The listing builds one solid part. Answer for the finished solid, in the listing's coordinates (mm). Round coordinates to 2 decimals unless told otherwise and drop trailing zeros. Order: outer loops, then holes, each group sorted by start corner. A loop starts at its lowest first (then second) coordinate and runs counter-clockwise, first axis right, second up. Notation, with made-up numbers: (43, 74.5) - (102, 74.5) arc R29 cw to (102, 102.5) - close; hole circle Ø8 at (1, 70.25). An arc over 180 degrees is marked (long way). One line per item, written item: value. Start each with the question number.
1. Section C-C, the plane y = 2 is taken. Give the vertices of the cut face in (x, z).
2. Section D-D, the plane z = -35 is taken. Give the vertices of the cut face in (x, y).
3. Section B-B, the plane x = -55 is taken. Give the vertices of the cut face in (y, z).
4. Section A-A, the plane x = -280 is taken. Give the vertices of the cut face in (y, z).
5. For a pull along Z with two mould halves and no side action, classify faces 1 (the flat face through (-150, 4, 0)), 2 (the flat face through (-145, 0, -25)), 3 (the flat face through (-145, 4, -50)), 4 (the cylindrical face through (-276.451, 4.563, -16.846)) as released by +Z, released by -Z, zero draft, split by the parting line, or undercut.
6. Straight lines are drawn through the part: line 1 (Z direction, x = -280, y = 4.5); line 2 (Z direction, x = -97.5, y = 5.5); line 3 (Z direction, x = -250, y = 3). For each, find the intervals that lie inside material, in ascending order.
7. A flat-ended cylindrical pin translates along its axis: P1, Ø6.5, axis at x = -280, z = -15, coming from the +Y side (3 decimals). Find the tip coordinate at first contact, or state that the pin passes through.
Autodesk Inventor part; units mm, degrees
ref_plane "YZ Plane" through (0, 0, 0) normal (1, 0, 0) x (0, 1, 0)
ref_plane "XZ Plane" through (0, 0, 0) normal (0, 1, 0) x (-1, 0, 0)
ref_plane "XY Plane" through (0, 0, 0) normal (0, 0, 1) x (1, 0, 0)
sketch "Skizze1" plane through (0, 0, 0) normal (0, 1, 0) x (-1, 0, 0)
  line L0 (0, 0) -> (275, 0)
  line L1 (275, 0) -> (275, -50)
  line L2 (275, -50) -> (0, -50)
  line L3 (0, -50) -> (0, 0)
  line L4 (275, 0) -> (275, -25)
  line L5 (275, -25) -> (250, -25)
  circle A0 centre (250, -25) radius 15
  line L6 (275, -50) -> (295, -50)
  line L7 (295, -50) -> (295, 0)
  line L8 (295, 0) -> (275, 0)
  dimension "d0" = 275
  dimension "d1" = 50
  dimension "d2" = 25
  dimension "d3" = 30
  dimension "d18" = 20
extrude "Extrusion1" add sketch "Skizze1" along normal blind 9 contours L0 L1 L2 L3
sketch "Skizze2" plane through (0, 9, 0) normal (0, 1, 0) x (1, 0, 0)
  line L0 (0, 0) -> (0, 50)
  line L1 (0, 50) -> (-30, 50)
  line L2 (-30, 50) -> (-30, 35)
  line L3 (0, 0) -> (-55, 0)
  line L4 (-275, 0) -> (0, 0)
  line L5 (-55, 0) -> (-70, 0)
  line L6 (-70, 0) -> (-55, 0)
  line L7 (-55, 0) -> (-55, 15)
  dimension "d6" = 30
  dimension "d7" = 15
  dimension "d8" = 55
  dimension "d9" = 15
  dimension "d10" = 15
hole "Bohrung1" at (-55, 9, -15) at (-30, 9, -35) direction (0, -1, 0) diameter 10 depth 10 tip angle 118
extrude "Extrusion2" add sketch "Skizze1" along normal blind 9 contours L8 L7 L6 L1
sketch "Skizze3" plane through (0, 0, 0) normal (0, -1, 0) x (1, 0, 0)
  line L0 (0, -50) -> (-295, -50)
  line L1 (-295, -50) -> (-280, -50)
  line L2 (-280, -50) -> (-280, -35)
  line L3 (-280, -35) -> (-280, -15)
  line L4 (-280, -15) -> (-280, 0)
  line L5 (-295, 0) -> (0, 0)
  dimension "d21" = 15
  dimension "d22" = 15
  dimension "d23" = 20
hole "Bohrung2" at (-280, 0, -15) at (-280, 0, -35) direction (0, 1, 0) diameter 8 depth 9 tip angle 118
sketch "Skizze4" plane through (0, 0, 0) normal (0, -1, 0) x (1, 0, 0)
  line L0 (-97.5, -25) -> (-97.5, 0)
  line L1 (-97.5, 0) -> (-97.5, -10)
  line L2 (-97.5, -10) -> (-97.5, -40)
  line L3 (0, 0) -> (0, -50)
  point P0 (-250, -25)
  point P1 (-223.5, -37.5)
  point P2 (-223.5, -12.5)
  point P3 (-138.5, -37.5)
  point P4 (-138.5, -12.5)
  dimension "d45" = 10
  dimension "d46" = 30
  dimension "d47" = 97.5
hole "Bohrung3" at (-97.5, 0, -40) at (-97.5, 0, -10) direction (0, 1, 0) diameter 5 end through all
properties part number "Lagerstuetze_Sensor" material "Holz (Birke)"
Answer list:
1. outline: (-295, -50) - (0, -50) - (0, 0) - (-295, 0) - close; hole circle Ø8 at (-280, -35); hole circle Ø8 at (-280, -15); hole circle Ø30 at (-250, -25); hole circle Ø5 at (-97.5, -40); hole circle Ø5 at (-97.5, -10); hole circle Ø10 at (-55, -15); hole circle Ø10 at (-30, -35)
2. outline: (-295, 0) - (-284, 0) - (-284, 9) - (-295, 9) - close; (-276, 0) - (-261.18, 0) - (-261.18, 9) - (-276, 9) - close; (-238.82, 0) - (-35, 0) - (-35, 9) - (-238.82, 9) - close; (-25, 0) - (0, 0) - (0, 9) - (-25, 9) - close
3. outline: (0, -50) - (9, -50) - (9, -20) - (0, -20) - close; (0, -10) - (9, -10) - (9, 0) - (0, 0) - close
4. outline: (0, -50) - (9, -50) - (9, -39) - (0, -39) - close; (0, -31) - (9, -31) - (9, -19) - (0, -19) - close; (0, -11) - (9, -11) - (9, 0) - (0, 0) - close
5. face 1: released by +Z
5. face 2: zero draft
5. face 3: released by -Z
5. face 4: undercut
6. line 1: z = -50 to -39, -31 to -19, -11 to 0
6. line 2: z = -50 to -42.5, -37.5 to -12.5, -7.5 to 0
6. line 3: z = -50 to -40, -10 to 0
7. P1: passes through
